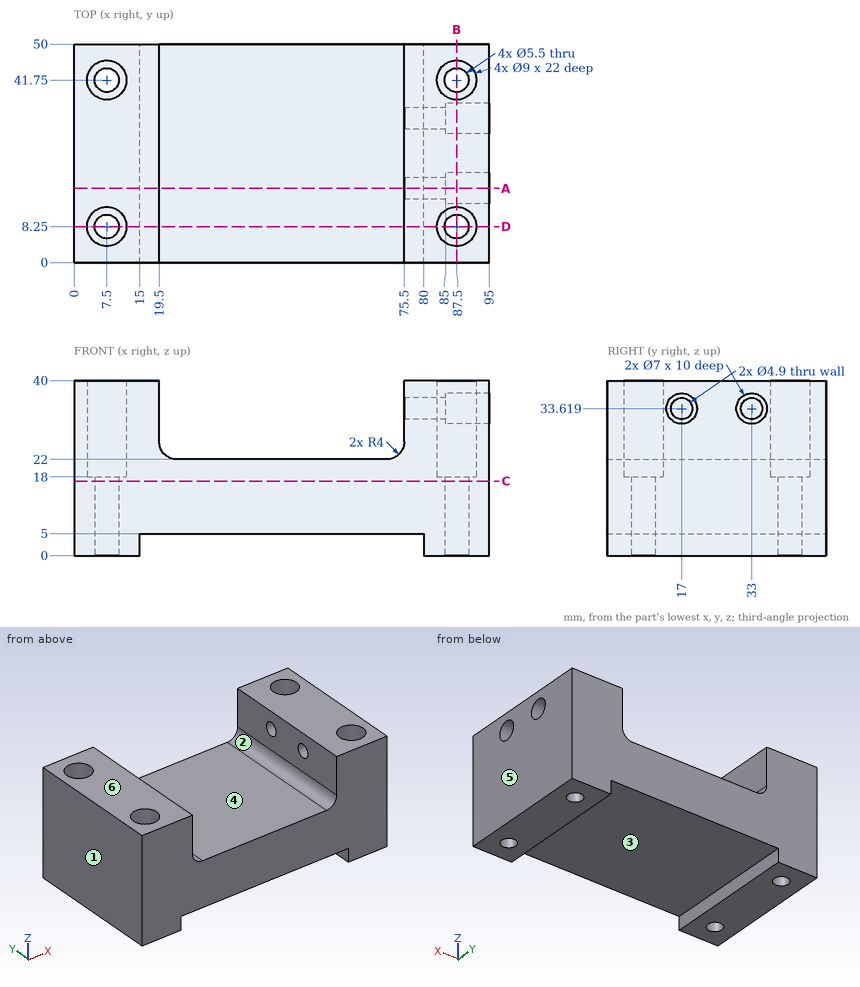
Print and shaded views of the part. All mm, measured from the part's lowest x, y and z. A direction names the side the tool comes from. Give positions to 0.01 mm unless a question says otherwise; leave off trailing zeros. Loops run counter-clockwise (first coordinate to the right, second up) from the corner with the lowest first, then second, coordinate; pieces in that order, holes last.
1) Tool access for the marked faces 1, 2 and 3: list every direction of +Z, -Z, +X, -X, +Y, -Y with a clear straight run to the whole face (end or side of a thin tool).
2) Pull direction X, two halves, no side cores. Call the marked faces 4, 5 and 6: +X half, -X half, draft (parallel to the pull), parting line (faces both ways), or undercut.
3) Saw through at D-D (y = 8.25). Count the separate pieces of the cut face and the enclosed holes in it, plus the area to 3 significant figures.
4) Saw through at C-C (z = 17). Write the cut outline in (x, y), plus the area to 4 significant figures.
5) Wall check: line 1 (Y direction, x = 87.5, z = 4.5); line 2 (X direction, y = 8.5, z = 6); line 3 (Y direction, x = 79, z = 32.5). Give the ranges that are in metal, low to high.
6) Flat gauge pins, fed straight in: pin 1 Ø1.5 at (x, y) = (30, 14.5) entering from -Z; pin 2 Ø7 at (x, y) = (87.5, 41.75) entering from +Z; pin 3 Ø4 at (y, z) = (33, 33.62) entering from +X; pin 4 Ø6 at (x, z) = (35.5, 27.5) entering from -Y. Where does each tip first touch, or does it go through?
7) Saw through at A-A (y = 17). Write the cut outline in (x, z).
8) Saw through at B-B (x = 87.5). Write the cut outline in (y, z).
Answer block:
1. face 1: +Z, -Z, -X, +Y, -Y
1. face 2: +Z, +Y, -Y
1. face 3: -Z, +Y, -Y
2. face 4: undercut
2. face 5: +X half
2. face 6: draft
3. separate pieces: 3
3. enclosed holes: 0
3. area: 1,880 mm2
4. outline: (0, 0) - (95, 0) - (95, 50) - (0, 50) - close; hole circle Ø5.5 at (7.5, 8.25); hole circle Ø5.5 at (7.5, 41.75); hole circle Ø5.5 at (87.5, 8.25); hole circle Ø5.5 at (87.5, 41.75)
4. area: 4,655 mm2
5. line 1: y = 0 to 5.5, 11 to 39, 44.5 to 50
5. line 2: x = 0 to 4.76, 10.24 to 84.76, 90.24 to 95
5. line 3: y = 0 to 14.82, 19.18 to 30.82, 35.18 to 50
6. pin 1: stops at z = 5
6. pin 2: stops at z = 18
6. pin 3: stops at x = 19.5
6. pin 4: passes through
7. outline: (0, 0) - (15, 0) - (15, 5) - (80, 5) - (80, 0) - (95, 0) - (95, 30.12) - (85, 30.12) - (85, 31.17) - (75.5, 31.17) - (75.5, 26) arc R4 cw to (71.5, 22) - (23.5, 22) arc R4 cw to (19.5, 26) - (19.5, 40) - (0, 40) - close; (75.5, 36.07) - (85, 36.07) - (85, 37.12) - (95, 37.12) - (95, 40) - (75.5, 40) - close
8. outline: (0, 0) - (5.5, 0) - (5.5, 18) - (3.75, 18) - (3.75, 40) - (0, 40) - close; (11, 0) - (39, 0) - (39, 18) - (37.25, 18) - (37.25, 40) - (12.75, 40) - (12.75, 18) - (11, 18) - close; (44.5, 0) - (50, 0) - (50, 40) - (46.25, 40) - (46.25, 18) - (44.5, 18) - close; hole circle Ø7 at (17, 33.62); hole circle Ø7 at (33, 33.62)
